Autodesk Inventor part; units mm, degrees
ref_plane "YZ Plane" through (0, 0, 0) normal (1, 0, 0) x (0, 1, 0)
ref_plane "XZ Plane" through (0, 0, 0) normal (0, 1, 0) x (-1, 0, 0)
ref_plane "XY Plane" through (0, 0, 0) normal (0, 0, 1) x (1, 0, 0)
sketch "Skizze2" plane through (0, 0, 0) normal (0, 0, 1) x (1, 0, 0)
  line L0 (0, -0.5) -> (0, 3)
  line L1 (-12, 0) -> (72, 0)
  line L2 (0, 0) -> (4, 0)
  line L3 (4, 1.5) -> (0, 1.5)
  line L4 (0, 1.5) -> (0, 0)
  line L5 (4, 0) -> (55, 0)
  line L6 (55, 1.5) -> (55, 2.5)
  line L7 (55, 2.5) -> (4, 2.5)
  line L8 (4, 2.5) -> (4, 1.5)
  line L9 (55, 0) -> (60, 0)
  line L10 (60, 0) -> (60, 1.5)
  line L11 (60, 1.5) -> (55, 1.5)
  dimension "d0" = 3
  dimension "d1" = 5
  dimension "d2" = 4
  dimension "d3" = 5
  dimension "d4" = 60
revolve "Umdrehung1" add sketch "Skizze2" angle 360 about axis through (-10, 0, 0) along (1, 0, 0)
thread "Gewinde1"
thread "Gewinde2"
chamfer "Fase1" distance 0.5 angle 45 2 edges at (60, -1.5, 0) (0, -1.5, 0)
properties part number "Kolbenstange"
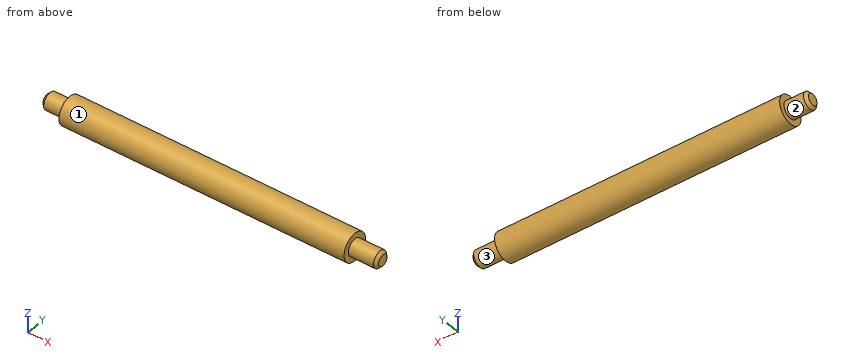
Model file for the job. Use its own axes, mm. Face numbers are marked on the shaded views. A direction names the side the tool comes from. Give positions to 0.01 mm unless a question says otherwise; leave off trailing zeros. Write each loop counter-clockwise with the first axis right and the second up, starting at its lowest first coordinate (ties: lowest second). Pieces come first, ordered by that corner, then holes. Notation, with made-up numbers: (14, 70) -> (52, 70) arc R13 cw to (52, 85) -> close; hole circle Ø6 at (-12.75, 7.5). An arc over 180 degrees is marked (long way). Use CSV: the item, a comma, the result in double quotes. Start each with the question number.
1) Cut at A-A on z = 0. List the corners of the cut face in (x, y), plus the area to 4 significant figures.
2) Pin check, flat tips, straight feed: P1, Ø1.5, axis at y = -1, z = 0.5, coming from the -X side; P2, Ø1.5, axis at x = 25.5, z = -1.5, coming from the +Y side. Stop position of each tip, or through.
3) Drill centre lines: L1, parallel to Y at x = 54.5, z = -0.2; L2, parallel to X at y = 0.15, z = 2.1. Where is each one in solid material? Low to high.
4) Tool access for the marked faces 1, 2 and 3: list every direction of +Z, -Z, +X, -X, +Y, -Y with a clear straight run to the whole face (end or side of a thin tool).
5) Cut at C-C on x = 32.5. List the corners of the cut face in (y, z).
Final values:
1,outline,"(0, -1) -> (0.5, -1.5) -> (4, -1.5) -> (4, -2.5) -> (55, -2.5) -> (55, -1.5) -> (59.5, -1.5) -> (60, -1) -> (60, 1) -> (59.5, 1.5) -> (55, 1.5) -> (55, 2.5) -> (4, 2.5) -> (4, 1.5) -> (0.5, 1.5) -> (0, 1) -> close"
1,area,"281.5 mm2"
2,P1,"stops at x = 0"
2,P2,"stops at y = 2.38"
3,L1,"y = -2.49 to 2.49"
3,L2,"x = 4 to 55"
4,face 1,"+X, -X"
4,face 2,"-X"
4,face 3,"+X"
5,outline,"circle Ø5 at (0, 0)"
